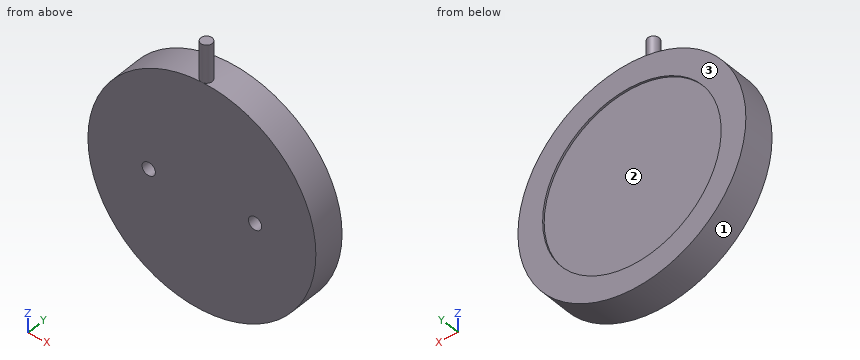
```python
from build123d import *

# Parameters (mm, degrees)
SKETCH_1_R          = 30
EXTRUDE_1_DEPTH     = 8.5
SKETCH_2_R          = 23.5
CUT_EXTRUDE_1_DEPTH = 0.5
SKETCH_3_R          = 1.5
EXTRUDE_2_DEPTH     = 15
SKETCH_4_R          = 1.75
CUT_EXTRUDE_2_DEPTH = 3


with BuildPart() as part:
    # 草图1 → 凸台-拉伸1 (new body)
    with BuildSketch(Plane(origin=(0, 0, 0), x_dir=(1, 0, 0), z_dir=(0, 1, 0))):
        Circle(SKETCH_1_R)
    extrude(amount=EXTRUDE_1_DEPTH)

    # 草图2 → 切除-拉伸1 (cut)
    with BuildSketch(Plane(origin=(0, 8.5, 0), x_dir=(1, 0, 0), z_dir=(0, 1, 0))):
        Circle(SKETCH_2_R)
    extrude(amount=-CUT_EXTRUDE_1_DEPTH, mode=Mode.SUBTRACT)

    # 草图3 → 凸台-拉伸2 (add)
    with BuildSketch(Plane.XY.offset(25)):
        with Locations((0, 1.5)):
            Circle(SKETCH_3_R)
    extrude(amount=EXTRUDE_2_DEPTH)

    # 草图4 → 切除-拉伸2 (cut)
    with BuildSketch(Plane.XZ):
        with Locations((-14, 0)):
            Circle(SKETCH_4_R)
        with Locations((14, 0)):
            Circle(SKETCH_4_R)
    extrude(amount=-CUT_EXTRUDE_2_DEPTH, mode=Mode.SUBTRACT)


solid = part.part
```
Can you work these out from the model? Positions are in its coordinate system, mm. Face numbers are marked on the shaded views. Coordinates: 2 decimals unless noted, no trailing zeros. Order: outer loops, then holes, each group sorted by start corner. A loop starts at its lowest first (then second) coordinate and runs counter-clockwise, first axis right, second up.
1. I need wall thicknesses on line 1 (X direction, y = 8.1, z = 0); line 2 (Y direction, x = -12.5, z = 11); line 3 (Z direction, x = 14, y = 2.05). Which ranges of each line are inside material? Lowest first, please.
2. If we section it at C-C (x = 10): Please give me the cut outline in (y, z).
3. If we section it at B-B (z = 0): Please give me the cut outline in (x, y), then the cut area to 4 significant figures.
4. If we section it at A-A (y = 1.5): Please give me the cut outline in (x, z).
5. I'm going to push flat-ended pins straight in: pin 1 (1 mm diameter, centred on x = -14, z = 0.5, fed in from -Y); pin 2 (1.5 mm diameter, centred on y = 5, z = 5.5, fed in from -X); pin 3 (1 mm diameter, centred on x = 7, y = 1.5, fed in from -Z). Where does each tip first touch, or does it pass through?
6. Thinking about a two-plate mould opening in X: for the marked faces 1, 2 and 3, which applies, +X half, -X half, draft (parallel to the pull), parting line (faces both ways), or undercut?
7. If we section it at D-D (z = -11.5): Please give me the cut outline in (x, y), then the cut area to 3 significant figures.
Entries:
1. line 1: x = -30 to -23.5, 23.5 to 30
1. line 2: y = 0 to 8
1. line 3: z = -26.53 to -1.75, 1.75 to 26.53
2. outline: (0, -28.28) - (8.5, -28.28) - (8.5, -21.27) - (8, -21.27) - (8, 21.27) - (8.5, 21.27) - (8.5, 28.28) - (0, 28.28) - close
3. outline: (-30, 0) - (-15.75, 0) - (-15.75, 3) - (-12.25, 3) - (-12.25, 0) - (12.25, 0) - (12.25, 3) - (15.75, 3) - (15.75, 0) - (30, 0) - (30, 8.5) - (23.5, 8.5) - (23.5, 8) - (-23.5, 8) - (-23.5, 8.5) - (-30, 8.5) - close
3. area: 465.5 mm2
4. outline: (-1.5, 29.96) arc R30 ccw (long way) to (1.5, 29.96) - (1.5, 40) - (-1.5, 40) - close; hole circle Ø3.5 at (-14, 0); hole circle Ø3.5 at (14, 0)
5. pin 1: stops at y = 3
5. pin 2: stops at x = -29.62
5. pin 3: stops at z = -29.29
6. face 1: parting line
6. face 2: undercut
6. face 3: draft
7. outline: (-27.71, 0) - (27.71, 0) - (27.71, 8.5) - (20.49, 8.5) - (20.49, 8) - (-20.49, 8) - (-20.49, 8.5) - (-27.71, 8.5) - close
7. area: 451 mm2
